Source: CAD feature listing. Evaluate the final solid. Frame: model axes, mm. A direction names the side the tool comes from. Give positions to 0.01 mm unless a question says otherwise; leave off trailing zeros. Order: outer loops, then holes, each group sorted by start corner. A loop starts at its lowest first (then second) coordinate and runs counter-clockwise, first axis right, second up. Notation, with made-up numbers: M 54.5,78 L 68.5,78 A17 cw 68.5,89 Z; hole C 35,35 d1. An arc over 180 degrees is marked long. Answer as a JSON object with one key per item and string values. Group by question number.
1. Section query B-B (z = 32). Output: boundary loops of the cut face in (x, y).
2. Section query A-A (x = -70). Output: boundary loops of the cut face in (y, z), plus the area to 3 significant figures.
3. Material intervals for L1, parallel to Y at x = -21.5, z = 70.5; L2, parallel to X at y = 53, z = -1, sorted ascending. Write a range as [from, to].
4. Set-up query: faces 1 (the flat face through (-9.75, 78, 0)), 2 (the flat face through (0, 40, -15)), 3 (the flat face through (15, 40, 0)). Return all of +Z, -Z, +X, -X, +Y, -Y with unobstructed straight access to the full face (end or side cutting, diameter ignored); none if empty.
5. Pin query (flat end, axial travel): P1, Ø12, axis at x = -24, y = 73, coming from the +Z side; P2, Ø3, axis at y = 77.5, z = 5, coming from the +X side; P3, Ø3, axis at x = 6.5, y = 56, coming from the +Z side; P4, Ø24, axis at y = 44, z = 0.5, coming from the +X side. Return the tip coordinate at first contact, or that it passes through.
from build123d import *

# Parameters (mm, degrees)
SKETCH1_W           = 170
SKETCH1_H           = 170
BOSS_EXTRUDE1_DEPTH = 5
SKETCH2_W           = 30
SKETCH2_H           = 30
BOSS_EXTRUDE2_DEPTH = 70
SKETCH3_W           = 19.5
SKETCH3_H           = 19.5
BOSS_EXTRUDE3_DEPTH = 6


with BuildPart() as part:
    # Sketch1 → Boss-Extrude1 (new body)
    with BuildSketch(Plane(origin=(0, 0, 0), x_dir=(1, 0, 0), z_dir=(0, 1, 0))):
        Rectangle(SKETCH1_W, SKETCH1_H)
    extrude(amount=BOSS_EXTRUDE1_DEPTH)

    # Sketch2 → Boss-Extrude2 (add)
    with BuildSketch(Plane(origin=(0, 5, 0), x_dir=(1, 0, 0), z_dir=(0, 1, 0))):
        Rectangle(SKETCH2_W, SKETCH2_H)
    extrude(amount=BOSS_EXTRUDE2_DEPTH)

    # Sketch3 → Boss-Extrude3 (add)
    with BuildSketch(Plane(origin=(0, 75, 0), x_dir=(1, 0, 0), z_dir=(0, 1, 0))):
        Rectangle(SKETCH3_W, SKETCH3_H)
    extrude(amount=BOSS_EXTRUDE3_DEPTH)


solid = part.part
Answer sheet:
{
 "1": {"outline": "M -85,0 L 85,0 L 85,5 L -85,5 Z"},
 "2": {"outline": "M 0,-85 L 5,-85 L 5,85 L 0,85 Z", "area": "850 mm^2"},
 "3": {"L1": "[0, 5]", "L2": "[-15, 15]"},
 "4": {"face 1": "+Z, -Z, -X, +Y", "face 2": "-Z, +X, -X, +Y", "face 3": "+Z, -Z, +X, +Y"},
 "5": {"P1": "through", "P2": "x = 9.75", "P3": "z = 15", "P4": "x = 15"}
}
